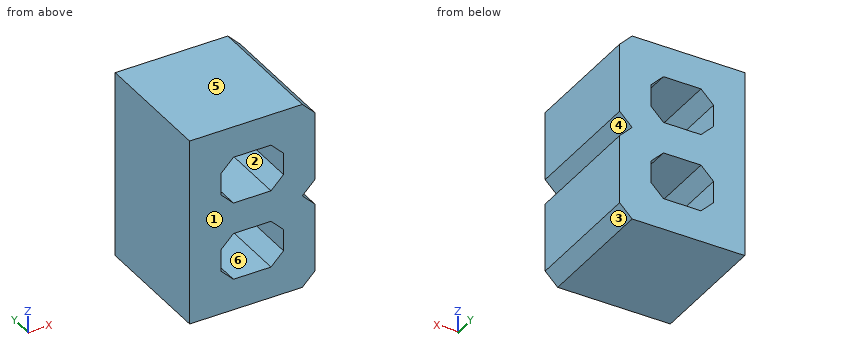
from build123d import *

# Parameters (mm, degrees)
F0_W     = 10
F0_H     = 7.5
F1_DEPTH = 20
F2_SIZE  = 2
F4_DEPTH = 25


# Not quite as in the source:
# - a feature names something its author has since deleted; it is built from what else it names


with BuildPart() as f1:
    # F0 (on Front) → F1 (new body)
    with BuildSketch(Plane.XZ):
        Polygon((20, 30), (0, 30), (0, 0), (20, 0), (20, 15), align=None)
        with Locations((10, 8.75)):
            Rectangle(F0_W, F0_H, mode=Mode.SUBTRACT)
        with Locations((10, 21.25)):
            Rectangle(F0_W, F0_H, mode=Mode.SUBTRACT)
    extrude(amount=F1_DEPTH)

    # F2
    f2_edges = [f1.edges().sort_by_distance(p)[0] for p in [
        (20, -10, 30),
        (5, -10, 17.5),
        (5, -10, 25),
        (5, -10, 12.5),
        (5, -10, 5),
        (15, -10, 25),
        (15, -10, 17.5),
        (15, -10, 12.5),
        (15, -10, 5),
        (20, -10, 0),
    ]]
    chamfer(f2_edges, length=F2_SIZE)

    # F3 (on face) → F4 (cut)
    with BuildSketch(Plane.XZ.offset(20)):
        Polygon((20, 13), (20, 15), (18, 15), align=None)
        Polygon((18, 15), (20, 15), (20, 17), align=None)
    extrude(amount=-F4_DEPTH, mode=Mode.SUBTRACT)


solid = f1.part
Can you work these out from the model? Positions are in its coordinate system, mm. Face numbers are marked on the shaded views. A direction names the side the tool comes from. Give positions to 0.01 mm unless a question says otherwise; leave off trailing zeros. Order: outer loops, then holes, each group sorted by start corner. A loop starts at its lowest first (then second) coordinate and runs counter-clockwise, first axis right, second up. Notation, with made-up numbers: M 11.5,-9.75 L 67.5,-9.75 A21 cw 67.5,14.25 Z; hole C 3,4 d5. An arc over 180 degrees is marked long. Use one line per item in the form item = value. Start each with the question number.
Item 1: We'd pull the mould along Z, two halves only. Please class the marked faces 1, 2 and 3: +Z half, -Z half, draft (parallel to the pull), parting line (faces both ways), or undercut.
Item 2: If we section it at D-D (z = 13.5): Write out the boundary of the cut face in (x, y).
Item 3: If I drill on line 1 along Z through (x, y) = (8.75, -13); line 2 along Z through (x, y) = (14.75, -9.5); line 3 along X through (y, z) = (-6, 9.75), over which ranges is the centre line in solid material (lowest first)?
Item 4: If we section it at B-B (x = 12.25): Write out the boundary of the cut face in (y, z), then the cut area to 3 significant figures.
Item 5: For the marked faces 4, 5 and 6, which set-ups out of +Z, -Z, +X, -X, +Y, -Y let a thin tool reach every point of the face, with its end or its side?
Item 6: If we section it at C-C (y = -9.25): Write out the boundary of the cut face in (x, z), then the cut area to 3 significant figures.
Item 7: If we section it at A-A (z = 9.5): Write out the boundary of the cut face in (x, y).
Outcome:
q1.face_1 = draft
q1.face_2 = undercut
q1.face_3 = -Z half
q2.outline = M 0,-20 L 19.5,-20 L 19.5,0 L 0,0 Z
q3.line_1 = 0 to 5, 12.5 to 17.5, 25 to 30
q3.line_2 = 0 to 6.75, 10.75 to 19.25, 23.25 to 30
q3.line_3 = 0 to 5, 15 to 20
q4.outline = M -20,0 L 0,0 L 0,5 L -20,5 Z; M -20,12.5 L 0,12.5 L 0,17.5 L -20,17.5 Z; M -20,25 L 0,25 L 0,30 L -20,30 Z
q4.area = 300 mm2
q5.face_4 = +X, +Y, -Y
q5.face_5 = +Z, +X, -X, +Y, -Y
q5.face_6 = +Y, -Y
q6.outline = M 0,0 L 18,0 L 20,2 L 20,13 L 18,15 L 20,17 L 20,28 L 18,30 L 0,30 Z; hole M 5,7 L 7,5 L 13,5 L 15,7 L 15,10.5 L 13,12.5 L 7,12.5 L 5,10.5 Z; hole M 5,19.5 L 7,17.5 L 13,17.5 L 15,19.5 L 15,23 L 13,25 L 7,25 L 5,23 Z
q6.area = 458 mm2
q7.outline = M 0,-20 L 5,-20 L 5,0 L 0,0 Z; M 15,-20 L 20,-20 L 20,0 L 15,0 Z
